from build123d import *

# Parameters (mm, degrees)
SKETCH_1_W      = 40
SKETCH_1_H      = 75
SKETCH_1_R      = 1.65
SKETCH_1_R_2    = 13.5
EXTRUDE_1_DEPTH = 5
FILLET_1_R      = 3


with BuildPart() as part:
    # 草图1 → 凸台-拉伸1 (new body)
    with BuildSketch(Plane(origin=(0, 0, 0), x_dir=(1, 0, 0), z_dir=(0, 1, 0))):
        with Locations((0, 17.5)):
            Rectangle(SKETCH_1_W, SKETCH_1_H)
        with Locations((-16, 16)):
            Circle(SKETCH_1_R, mode=Mode.SUBTRACT)
        with Locations((16, 16)):
            Circle(SKETCH_1_R, mode=Mode.SUBTRACT)
        with Locations((16, -16)):
            Circle(SKETCH_1_R, mode=Mode.SUBTRACT)
        with Locations((-16, -16)):
            Circle(SKETCH_1_R, mode=Mode.SUBTRACT)
        with Locations((0, 33.6)):
            Circle(SKETCH_1_R_2, mode=Mode.SUBTRACT)
    extrude(amount=EXTRUDE_1_DEPTH)

    # 圆角1
    fillet_1_edges = [part.edges().sort_by_distance(p)[0] for p in [
        (20, 2.5, 20),
        (-20, 2.5, 20),
        (-20, 2.5, -55),
        (20, 2.5, -55),
    ]]
    fillet(fillet_1_edges, radius=FILLET_1_R)


solid = part.part
Work out the finished part from the listing and answer in its coordinate system (mm). Give positions to 0.01 mm unless a question says otherwise; leave off trailing zeros. Order: outer loops, then holes, each group sorted by start corner. A loop starts at its lowest first (then second) coordinate and runs counter-clockwise, first axis right, second up. Notation, with made-up numbers: (-29.5, 68.5) - (12.5, 68.5) arc R7 ccw to (12.5, 76.5) - close; hole circle Ø6 at (73.25, 80.5). An arc over 180 degrees is marked (long way). Answer as CSV lines item,"result". Start each with the question number.
Q1. Find the intervals of material crossed by L1, parallel to X at y = 3.95, z = -16; L2, parallel to Z at x = 16, y = 3.55; L3, parallel to Z at x = -17, y = 3, in increasing order. Write a range as [from, to].
Q2. The mould has two halves that part along X. Classify faces 1 (the face through (-19.14, 2.54, -54.1)), 2 (the face through (0, 2, -55)), 3 (the face through (17.574, 2.465, -16.496)): +X half, -X half, draft (parallel to the pull), parting line (faces both ways), or undercut.
Q3. The part is cut by section A-A (x = 0). Write down the section's boundary in (y, z).
Q4. The part is cut by section B-B (y = 4.05). Write down the section's boundary in (x, z).
Q5. The part is cut by section D-D (x = -16). Write down the section's boundary in (y, z), then the cut area to 3 significant figures.
Q6. Given pin 1 Ø4 at (x, z) = (10.5, 6.5) entering from -Y; pin 2 Ø3 at (x, z) = (-16, 16) entering from -Y, each flat-ended and moving along its own axis, determine where each tip first touches the part or whether it passes through.
Q7. The part is cut by section C-C (z = -16). Write down the section's boundary in (x, y), then the cut area to 3 significant figures.
Check result:
1,L1,"x = [-20, -17.65], [-14.35, 14.35], [17.65, 20]"
1,L2,"z = [-55, -17.65], [-14.35, 14.35], [17.65, 20]"
1,L3,"z = [-55, -17.31], [-14.69, 14.69], [17.31, 20]"
2,face 1,"-X half"
2,face 2,"draft"
2,face 3,"undercut"
3,outline,"(0, -55) - (5, -55) - (5, -47.1) - (0, -47.1) - close; (0, -20.1) - (5, -20.1) - (5, 20) - (0, 20) - close"
4,outline,"(-20, -52) arc R3 ccw to (-17, -55) - (17, -55) arc R3 ccw to (20, -52) - (20, 17) arc R3 ccw to (17, 20) - (-17, 20) arc R3 ccw to (-20, 17) - close; hole circle Ø3.3 at (-16, -16); hole circle Ø3.3 at (-16, 16); hole circle Ø27 at (0, -33.6); hole circle Ø3.3 at (16, -16); hole circle Ø3.3 at (16, 16)"
5,outline,"(0, -55) - (5, -55) - (5, -17.65) - (0, -17.65) - close; (0, -14.35) - (5, -14.35) - (5, 14.35) - (0, 14.35) - close; (0, 17.65) - (5, 17.65) - (5, 20) - (0, 20) - close"
5,area,"342 mm²"
6,pin 1,"stops at y = 0"
6,pin 2,"passes through"
7,outline,"(-20, 0) - (-17.65, 0) - (-17.65, 5) - (-20, 5) - close; (-14.35, 0) - (14.35, 0) - (14.35, 5) - (-14.35, 5) - close; (17.65, 0) - (20, 0) - (20, 5) - (17.65, 5) - close"
7,area,"167 mm²"
